Design review of the part built by this model. Coordinates are the model's own, in mm. Round coordinates to 2 decimals unless told otherwise and drop trailing zeros. Loops run counter-clockwise (first coordinate to the right, second up) from the corner with the lowest first, then second, coordinate; pieces in that order, holes last. Notation, with made-up numbers: M 52.25,-34 L 91.25,-34 A25 cw 91.25,-4 Z; hole C 72,77 d7. An arc over 180 degrees is marked long. Use a Markdown table: item, result.
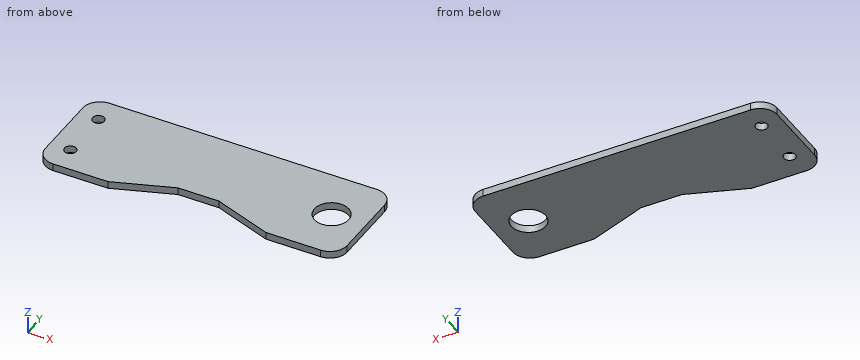
from build123d import *

# Parameters (mm, degrees)
CROQUIS1_W              = 88
CROQUIS1_H              = 30
CROQUIS1_R              = 1.7
SALIENTE_EXTRUIR1_DEPTH = 2.11
CROQUIS6_R              = 5
CORTAR_EXTRUIR2_DEPTH   = 2.11
CORTAR_EXTRUIR3_DEPTH   = 2.11
REDONDEO1_R             = 5


with BuildPart() as part:
    # Croquis1 → Saliente-Extruir1 (new body)
    with BuildSketch(Plane.XY):
        with Locations((36.708826457, -6.405767977)):
            Rectangle(CROQUIS1_W, CROQUIS1_H)
        with Locations((-1.37457934, 1.094232023)):
            Circle(CROQUIS1_R, mode=Mode.SUBTRACT)
        with Locations((-1.37457934, -13.905767977)):
            Circle(CROQUIS1_R, mode=Mode.SUBTRACT)
    extrude(amount=SALIENTE_EXTRUIR1_DEPTH)

    # Croquis6 → Cortar-Extruir2 (cut)
    with BuildSketch(Plane.XY.offset(2.11)):
        with Locations((70.708826457, -6.405767977)):
            Circle(CROQUIS6_R)
    extrude(amount=-CORTAR_EXTRUIR2_DEPTH, mode=Mode.SUBTRACT)

    # Croquis7 → Cortar-Extruir3 (cut)
    with BuildSketch(Plane.XY.offset(2.11)):
        Polygon((13.708826457, -21.405767977), (30.708826457, -15.218273994), (42.708826457, -15.218273994), (59.708826457, -21.405767977), align=None)
    extrude(amount=-CORTAR_EXTRUIR3_DEPTH, mode=Mode.SUBTRACT)

    # Redondeo1
    redondeo1_edges = [part.edges().sort_by_distance(p)[0] for p in [
        (80.708826457, 8.594232023, 1.055),
        (80.708826457, -21.405767977, 1.055),
        (-7.291173543, -21.405767977, 1.055),
        (-7.291173543, 8.594232023, 1.055),
    ]]
    fillet(redondeo1_edges, radius=REDONDEO1_R)


solid = part.part
1. Take a section at D-D on x = 47. Give the boundary of the cut face in (y, z).
Check values:
| item | result |
|---|---|
| outline | M -16.78,0 L 8.59,0 L 8.59,2.11 L -16.78,2.11 Z |
2. Insertion check: pin 1 (1.1 mm diameter, centred on x = 36.5, z = 1, fed in from -Y). The pin has a flat end and moves straight along its axis. Give the tip position at first contact, or say it passes through.
Check values:
| item | result |
|---|---|
| pin 1 | stops at y = -15.22 |
3. Wall thickness on line 1 along X through (y, z) = (-9, 0.45); line 2 along X through (y, z) = (-3.25, 1.6); line 3 along Y through (x, z) = (41.5, 1.8): over which ranges is each line inside the solid? List them lowest first. Write a range as from..to.
Check values:
| item | result |
|---|---|
| line 1 | x = -7.29..66.43, 74.98..80.71 |
| line 2 | x = -7.29..66.83, 74.59..80.71 |
| line 3 | y = -15.22..8.59 |
4. Take a section at A-A on y = 2. Give the boundary of the cut face in (x, z), and give its area (3 significant figures).
Check values:
| item | result |
|---|---|
| outline | M -7.29,0 L -2.81,0 L -2.81,2.11 L -7.29,2.11 Z; M 0.06,0 L 80.71,0 L 80.71,2.11 L 0.06,2.11 Z |
| area | 180 mm² |
5. Take a section at C-C on z = 1.3. Give the boundary of the cut face in (x, y).
Check values:
| item | result |
|---|---|
| outline | M -7.29,-16.41 A5 ccw -2.29,-21.41 L 13.71,-21.41 L 30.71,-15.22 L 42.71,-15.22 L 59.71,-21.41 L 75.71,-21.41 A5 ccw 80.71,-16.41 L 80.71,3.59 A5 ccw 75.71,8.59 L -2.29,8.59 A5 ccw -7.29,3.59 Z; hole C -1.37,-13.91 d3.4; hole C -1.37,1.09 d3.4; hole C 70.71,-6.41 d10 |
6. Take a section at B-B on x = 66.5. Give the boundary of the cut face in (y, z).
Check values:
| item | result |
|---|---|
| outline | M -21.41,0 L -9.1,0 L -9.1,2.11 L -21.41,2.11 Z; M -3.71,0 L 8.59,0 L 8.59,2.11 L -3.71,2.11 Z |
